Autodesk Inventor part; units mm, degrees
ref_plane "YZ Plane" through (0, 0, 0) normal (1, 0, 0) x (0, 1, 0)
ref_plane "XZ Plane" through (0, 0, 0) normal (0, 1, 0) x (-1, 0, 0)
ref_plane "XY Plane" through (0, 0, 0) normal (0, 0, 1) x (1, 0, 0)
sketch "Эскиз1" plane through (0, 0, 0) normal (0, 1, 0) x (-1, 0, 0)
  line L0 (-52.75, 16.25) -> (52.75, 16.25)
  line L1 (52.75, 16.25) -> (52.75, -16.25)
  line L2 (52.75, -16.25) -> (-52.75, -16.25)
  line L3 (-52.75, -16.25) -> (-52.75, 16.25)
  line L4 (-52.75, 16.25) -> (52.75, -16.25) construction
  line L5 (52.75, 16.25) -> (-52.75, -16.25) construction
  line L6 (-42.75, -14.25) -> (0, -14.25)
  line L7 (42.75, -14.25) -> (42.75, -2.1082)
  line L8 (42.75, 14.25) -> (6.3246, 14.25)
  line L9 (-42.75, 14.25) -> (-42.75, -14.25)
  line L10 (52.75, -16.25) -> (36.5, 0) construction
  line L11 (36.5, 0) -> (52.75, 16.25) construction
  line L12 (47.75, -16.25) -> (47.75, 16.25) construction
  line L13 (0, -22.75) -> (0, 22.75) construction
  line L14 (0, -16.25) -> (0, -14.25) construction
  line L15 (0, 14.25) -> (0, 16.25) construction
  line L16 (0, -14.25) -> (42.75, 0)
  line L17 (42.75, 0) -> (0, 14.25)
  line L18 (42.75, -2.1082) -> (6.3246, -14.25)
  line L19 (42.75, 2.1082) -> (6.3246, 14.25)
  line L20 (42.75, -2.1082) -> (42.1175, -0.2108) construction
  line L21 (42.75, 2.1082) -> (42.1175, 0.2108) construction
  line L22 (42.75, -2.1082) -> (42.75, 2.1082) construction
  line L23 (42.75, 2.1082) -> (42.75, 14.25)
  line L24 (6.3246, -14.25) -> (42.75, -14.25)
  line L25 (0, -14.25) -> (6.3246, -14.25) construction
  line L26 (6.3246, 14.25) -> (0, 14.25) construction
  line L27 (0, 14.25) -> (-42.75, 14.25)
  point P0 (0, 0)
  point P1 (0, 0)
  dimension "d0" = 105.5
  dimension "d4" = 10
  dimension "d5" = 10
  dimension "d8" = 5
  dimension "d24" = 28.5
  dimension "d29" = 2
extrude "Выдавливание1" add sketch "Эскиз1" along normal blind 2
sketch "Эскиз2" plane through (0, 0, 0) normal (0, 1, 0) x (-1, 0, 0)
  line L0 (-42.75, -16.25) -> (-42.75, 16.25)
  line L1 (52.75, 16.25) -> (-52.75, 16.25)
  line L2 (-52.75, 16.25) -> (-52.75, -16.25)
  line L3 (0, -14.25) -> (-42.75, -14.25) construction
  line L4 (-40.75, -14.25) -> (-40.75, 14.25) construction
  line L5 (6.3246, 14.25) -> (42.75, 14.25) construction
  line L6 (-40.75, -14.25) -> (-26.5, -14.25) construction
  line L7 (-6.75, -14.25) -> (-6.75, -16.25)
  line L8 (-52.75, -16.25) -> (52.75, -16.25)
  line L9 (-6.75, -16.25) -> (-42.75, -16.25)
  line L10 (-42.75, 16.25) -> (-6.75, 16.25)
  line L11 (-6.75, 14.25) -> (-26.5, 14.25)
  line L12 (-6.75, 14.25) -> (-6.75, 16.25)
  arc A0 (-26.5, 14.25) -> (-26.5, -14.25) centre (-26.5, 0) ccw
  line L13 (-26.5, -14.25) -> (-6.75, -14.25)
  line L14 (-26.5, 14.25) -> (-40.75, 14.25) construction
  line L15 (-42.75, -14.25) -> (-42.75, 14.25)
  point P0 (0, 0)
  point P1 (42.75, -14.25)
  point P2 (-42.75, -16.25)
  dimension "d13" = 2
  dimension "d14" = 34
extrude "Выдавливание2" add sketch "Эскиз2" along normal blind 13 contours L0 L1 L12 L11 A0 L13 L7 L8
sketch "Эскиз3" plane through (0, 2, 0) normal (0, 1, 0) x (1, 0, 0)
  line L0 (-42.75, 14.25) -> (-52.75, 14.25)
  line L1 (-52.75, 14.25) -> (-52.75, 16.25)
  line L2 (-52.75, 16.25) -> (-42.75, 16.25)
  line L3 (-42.75, 16.25) -> (-42.75, 14.25)
  line L4 (-52.75, 16.25) -> (-52.75, -16.25) construction
  line L5 (-52.75, -16.25) -> (-42.75, -16.25)
  line L6 (-42.75, -16.25) -> (-42.75, -14.25)
  line L7 (-42.75, -14.25) -> (-52.75, -14.25)
  line L8 (-52.75, -14.25) -> (-52.75, -16.25)
  point P0 (0, 0)
  point P1 (-42.75, 14.25)
extrude "Выдавливание3" add sketch "Эскиз3" along normal blind 35
sketch "Эскиз4" plane through (-52.75, 0, 16.25) normal (0, 0, 1) x (1, 0, 0)
  line L0 (10, 37) -> (0, 37) construction
  line L1 (0, 37) -> (10, 37) construction
  line L2 (10, 37) -> (10, 27) construction
  line L3 (10, 27) -> (0, 27) construction
  line L4 (0, 27) -> (0, 37) construction
  line L5 (105.5, 0) -> (0, 0) construction
  line L6 (0, 0) -> (0, 37) construction
  line L7 (10, 37) -> (10, 2) construction
  line L8 (10, 2) -> (59.5, 2) construction
  line L9 (59.5, 2) -> (59.5, 13) construction
  line L10 (59.5, 13) -> (95.5, 13) construction
  line L11 (95.5, 13) -> (95.5, 2) construction
  line L12 (95.5, 2) -> (105.5, 2) construction
  line L13 (105.5, 2) -> (105.5, 0) construction
  line L14 (10, 2) -> (10, 37) construction
  line L15 (0, 0) -> (0, 37) construction
  line L16 (10, 27) -> (0, 37) construction
  line L17 (10, 37) -> (0, 27) construction
  circle A0 centre (5, 32) radius 0.5
  line L18 (59.5, 13) -> (69.5, 13) construction
  line L19 (69.5, 13) -> (69.5, 3) construction
  line L20 (69.5, 3) -> (59.5, 3) construction
  line L21 (59.5, 3) -> (59.5, 13) construction
  line L22 (69.5, 13) -> (59.5, 3) construction
  line L23 (59.5, 2) -> (59.5, 13) construction
  line L24 (59.5, 13) -> (69.5, 3) construction
  circle A1 centre (64.5, 8) radius 0.5
  line L25 (0, 37) -> (10, 37)
  point P0 (52.75, 0)
  dimension "d19" = 1
  dimension "d20" = 10
  dimension "d21" = 1
hole "Отверстие1" at (-47.75, 32, 16.25) at (11.75, 8, 16.25) direction (0, 0, -1) diameter 1 depth 16.25 countersink diameter 1.5 countersink angle 90
mirror "Зеркальное отражение1" about plane through (0, 0, 0) normal (0, 0, 1) of "Отверстие1"
sketch "Эскиз5" plane through (0, 2, 0) normal (0, 1, 0) x (1, 0, 0)
  line L0 (-42.75, 2.1082) -> (-6.3246, 14.25) construction
  line L1 (-6.3246, 14.25) -> (-42.75, 14.25) construction
  line L2 (-42.75, 14.25) -> (-52.75, 14.25) construction
  line L3 (-52.75, -14.25) -> (-52.75, 14.25) construction
  line L4 (-52.75, -16.25) -> (-52.75, -14.25) construction
  line L5 (-42.75, -16.25) -> (-52.75, -16.25) construction
  line L6 (-42.75, -14.25) -> (-42.75, -16.25) construction
  line L7 (-42.75, -14.25) -> (-6.3246, -14.25) construction
  line L8 (-6.3246, -14.25) -> (-42.75, -2.1082) construction
  line L9 (-42.75, -2.1082) -> (-42.75, -14.25) construction
  line L10 (-42.75, 14.25) -> (-42.75, 2.1082) construction
  line L11 (-42.75, 16.25) -> (-42.75, 14.25) construction
  line L12 (-42.75, 16.25) -> (6.75, 16.25) construction
  line L13 (6.75, 16.25) -> (42.75, 16.25) construction
  line L14 (42.75, 16.25) -> (52.75, 16.25) construction
  line L15 (52.75, 16.25) -> (52.75, -16.25) construction
  line L16 (52.75, -16.25) -> (42.75, -16.25) construction
  line L17 (42.75, 16.25) -> (42.75, -16.25) construction
  line L18 (-52.75, 14.25) -> (-52.75, 16.25) construction
  line L19 (-52.75, 16.25) -> (-42.75, 16.25) construction
  line L20 (-52.75, -14.25) -> (-42.75, -14.25) construction
  line L21 (6.75, -16.25) -> (-42.75, -16.25) construction
  line L22 (42.75, -16.25) -> (6.75, -16.25) construction
  line L23 (6.75, 14.25) -> (6.75, 16.25) construction
  line L24 (6.75, 14.25) -> (0, 14.25) construction
  line L25 (0, 14.25) -> (-42.75, 0) construction
  line L26 (-42.75, 0) -> (0, -14.25) construction
  line L27 (0, -14.25) -> (6.75, -14.25) construction
  line L28 (6.75, -14.25) -> (26.5, -14.25) construction
  arc A0 (26.5, -14.25) -> (26.5, 14.25) centre (26.5, 0) ccw construction
  line L29 (26.5, 14.25) -> (6.75, 14.25) construction
  line L30 (6.75, -16.25) -> (6.75, -14.25) construction
  line L31 (-6.3246, -14.25) -> (-42.75, -14.25) construction
  line L32 (-52.75, 14.25) -> (-42.75, -14.25) construction
  line L33 (-42.75, 14.25) -> (-52.75, -14.25) construction
  line L34 (42.75, 16.25) -> (52.75, 0) construction
  line L35 (52.75, -16.25) -> (52.75, 16.25) construction
  line L36 (52.75, 0) -> (42.75, -16.25) construction
  line L37 (-52.75, -16.25) -> (52.75, -16.25) construction
  line L38 (52.75, -16.25) -> (42.75, 0) construction
  line L39 (52.75, 16.25) -> (-52.75, 16.25) construction
  line L40 (42.75, 0) -> (52.75, 16.25) construction
  circle A1 centre (-47.75, 0) radius 0.5
  circle A2 centre (47.75, 8.125) radius 0.5
  circle A3 centre (47.75, -8.125) radius 0.5
  point P0 (0, 0)
  dimension "d37" = 1
hole "Отверстие2" at (-47.75, 2, 0) at (47.75, 2, -8.125) at (47.75, 2, 8.125) direction (0, -1, 0) diameter 1 end through all countersink diameter 1.5 countersink angle 90
properties part number "frame"
Part model, mm, in its own coordinate system. A direction names the side the tool comes from. Round coordinates to 2 decimals unless told otherwise and drop trailing zeros. Order: outer loops, then holes, each group sorted by start corner. A loop starts at its lowest first (then second) coordinate and runs counter-clockwise, first axis right, second up. Notation, with made-up numbers: M -36.5,30 L -16.5,30 A15 ccw -16.5,49 Z; hole C 82,-29 d3. An arc over 180 degrees is marked long. Put each result on its own line as item: value. Start each with the question number.
1. Drill centre lines: probe 1 along X at (y, z) = (8, -15); probe 2 along Z at (x, y) = (-45, 7.5); probe 3 along Y at (x, z) = (11.75, -15). Where is each one in solid material? Low to high. Write a range as [from, to].
2. Slice it at B-B on x = 25. List the corners of the cut face in (y, z), then the cut area to 3 significant figures.
3. Slice it at D-D on y = 5. List the corners of the cut face in (x, z).
4. Two-plate mould, pull along Z, no slides. Class faces 6 (the face through (-8, 1, -16.25)), 7 (the face through (-42.75, 1, 8)), 8 (the face through (52.75, 1, 0)): +Z half, -Z half, draft (parallel to the pull), parting line (faces both ways), or undercut.
5. Slice it at A-A on y = 35.5. List the corners of the cut face in (x, z).
6. Tool access for faces 1 (the face through (-42.75, 19, 15)), 2 (the face through (-32, 2, -5)), 3 (the face through (-24.792, 0.986, -8.094)), 4 (the face through (-48, 19, 14.25)), 5 (the face through (42.75, 7, 0)): list every direction of +Z, -Z, +X, -X, +Y, -Y with a clear straight run to the whole face (end or side of a thin tool).
7. Drop flat-ended pins along their axis: pin 1 (5 mm diameter, centred on x = 46.5, z = -3.5, fed in from +Y); pin 2 (3 mm diameter, centred on y = 13.5, z = -3, fed in from +X); pin 3 (1.6 mm diameter, centred on y = 14.5, z = -15.5, fed in from +X). Give the stop position or say it passes through.
8. Slice it at C-C on z = 10. List the corners of the cut face in (x, y).
Findings:
1. probe 1: [-52.75, -42.75], [6.75, 11.25], [12.25, 42.75]
1. probe 2: [-16.25, -14.25], [14.25, 16.25]
1. probe 3: [0, 7.5], [8.5, 13]
2. outline: M 0,-16.25 L 13,-16.25 L 13,-14.25 L 0,-14.25 Z; M 0,14.25 L 13,14.25 L 13,16.25 L 0,16.25 Z
2. area: 52.0 mm2
3. outline: M -52.75,-16.25 L -42.75,-16.25 L -42.75,-14.25 L -52.75,-14.25 Z; M -52.75,14.25 L -42.75,14.25 L -42.75,16.25 L -52.75,16.25 Z; M 6.75,-16.25 L 42.75,-16.25 L 42.75,16.25 L 6.75,16.25 L 6.75,14.25 L 26.5,14.25 A14.25 cw 26.5,-14.25 L 6.75,-14.25 Z
4. face 6: -Z half
4. face 7: undercut
4. face 8: draft
5. outline: M -52.75,-16.25 L -42.75,-16.25 L -42.75,-14.25 L -52.75,-14.25 Z; M -52.75,14.25 L -42.75,14.25 L -42.75,16.25 L -52.75,16.25 Z
6. face 1: +Z, -Z, +Y
6. face 2: +Y
6. face 3: +Y, -Y
6. face 4: -X, +Y
6. face 5: +Z, -Z, +X, +Y
7. pin 1: y = 2
7. pin 2: x = 42.75
7. pin 3: x = -42.75
8. outline: M -52.75,0 L -42.75,0 L -42.75,2 L -52.75,2 Z; M -19.07,0 L -12.75,0 L -12.75,2 L -19.07,2 Z; M 36.65,0 L 52.75,0 L 52.75,2 L 42.75,2 L 42.75,13 L 36.65,13 Z
